Input: part model. Units: mm. Frame: model coordinates. A direction names the side the tool comes from. Give positions to 0.01 mm unless a question says otherwise; leave off trailing zeros. Write each loop counter-clockwise with the first axis right and the second up, starting at its lowest first coordinate (ties: lowest second). Pieces come first, ordered by that corner, then holes. Notation, with made-up numbers: (-16, 33.25) - (-1, 33.25) arc R24 cw to (-1, 72.25) - close; hole circle Ø8 at (63, 7.25). An arc over 180 degrees is marked (long way). Answer as CSV lines item,"result".
```python
from build123d import *

# Parameters (mm, degrees)
CHAMFER1_SIZE = 0.5


with BuildPart() as part:
    # Sketch1 → Revolve1 (revolve)
    with BuildSketch(Plane(origin=(0, 0, 0), x_dir=(0, 0, -1), z_dir=(1, 0, 0)), mode=Mode.PRIVATE) as revolve1_sk:
        Polygon((0, 9.5), (0, 22.5), (110, 22.5), (110, 17.5), (109.5, 17), (64, 17), (64, 12.5), (63.5, 12), (4, 12), (4, 9), (0.5, 9), align=None)
    revolve(revolve1_sk.sketch.rotate(Axis((0, 0, 0), (0, 0, -1)), 90), axis=Axis((0, 0, 0), (0, 0, -1)))

    # Chamfer1
    chamfer1_edges = [part.edges().sort_by_distance(p)[0] for p in [
        (-22.5, 0, -110),
        (-22.5, 0, 0),
    ]]
    chamfer(chamfer1_edges, length=CHAMFER1_SIZE)


solid = part.part
```
Item 1: Cut plane D-D on z = -47.5. Return the cut outline in (x, y).
The answers:
outline,"circle Ø45 at (0, 0); hole circle Ø24 at (0, 0)"
Item 2: Cut plane C-C on z = -96.5. Return the cut outline in (x, y).
The answers:
outline,"circle Ø45 at (0, 0); hole circle Ø34 at (0, 0)"
Item 3: Mould query, pull axis X, two halves, no side actions, for faces 3 (the face through (-15, 10, -110)), 4 (the face through (10.382, 19.961, -55.763)), 5 (the face through (2, -9, -4)). Classes: +X half, -X half, draft (parallel to the pull), parting line (faces both ways), or undercut.
The answers:
face 3,"draft"
face 4,"parting line"
face 5,"undercut"
Item 4: Contact query for flat-ended pins moving along their axis: pin 1 (21.5 mm diameter, centred on x = 0, y = 0, fed in from -Z); pin 2 (2 mm diameter, centred on x = -0.5, z = -75.5, fed in from -Y); pin 3 (2 mm diameter, centred on x = 2.5, y = 11.5, fed in from -Z). Output: stop coordinate, or through.
The answers:
pin 1,"z = -4"
pin 2,"y = -22.5"
pin 3,"z = -64"
Item 5: Ray query, line 1 (Y direction, x = 0, z = -1.3); line 2 (X direction, y = 0.5, z = -60); line 3 (Y direction, x = 0, z = -98). Return the intervals inside material, ascending. Write a range as from..to.
The answers:
line 1,"-22.5..-9, 9..22.5"
line 2,"-22.49..-11.99, 11.99..22.49"
line 3,"-22.5..-17, 17..22.5"
Item 6: Reachability of faces 1 (the face through (-9, -9, -64)), 2 (the face through (-6.633, -6.083, -2.226)) from +Z, -Z, +X, -X, +Y, -Y: full face, straight path, thin tool, end or side. Return the list, or none.
The answers:
face 1,"-Z"
face 2,"+Z, -Z"
Item 7: Cut plane A-A on x = 0. Return the cut outline in (y, z).
The answers:
outline,"(-22.5, -109.5) - (-22, -110) - (-17.5, -110) - (-17, -109.5) - (-17, -64) - (-12.5, -64) - (-12, -63.5) - (-12, -4) - (-9, -4) - (-9, -0.5) - (-9.5, 0) - (-22, 0) - (-22.5, -0.5) - close; (9, -4) - (12, -4) - (12, -63.5) - (12.5, -64) - (17, -64) - (17, -109.5) - (17.5, -110) - (22, -110) - (22.5, -109.5) - (22.5, -0.5) - (22, 0) - (9.5, 0) - (9, -0.5) - close"
